Model file for the job. Use its own axes, mm. Face numbers are marked on the shaded views. A direction names the side the tool comes from. Round coordinates to 2 decimals unless told otherwise and drop trailing zeros. Write each loop counter-clockwise with the first axis right and the second up, starting at its lowest first coordinate (ties: lowest second). Pieces come first, ordered by that corner, then holes.
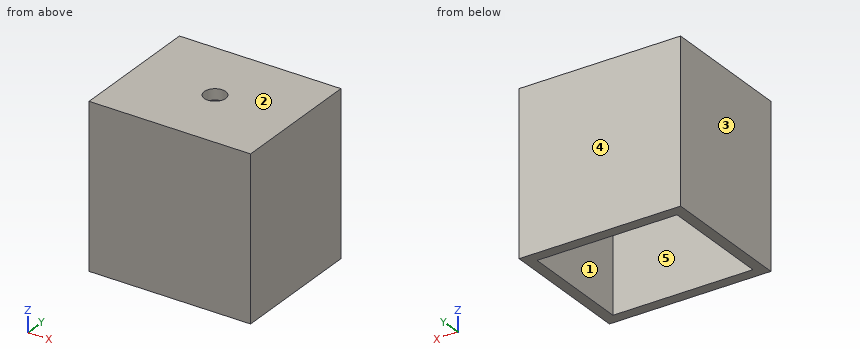
```python
from build123d import *

# Parameters (mm, degrees)
F0_W     = 15
F0_H     = 12.5
F1_DEPTH = 15
F2_T     = -1
F4_D     = 2


with BuildPart() as f1:
    # F0 (on Top) → F1 (new body)
    with BuildSketch(Plane.XY):
        Rectangle(F0_W, F0_H)
    extrude(amount=F1_DEPTH)

    # F2
    f2_openings = [f1.faces().sort_by_distance(p)[0] for p in [
        (0, 0, 0),
    ]]
    offset(amount=F2_T, openings=f2_openings)

    # F4 (through all)
    with Locations(Plane.XY.offset(15)):
        with Locations((0, 0)):
            Hole(F4_D / 2)


solid = f1.part
```
1) Wall check: probe 1 along Y at (x, z) = (3.75, 10.25); probe 2 along X at (y, z) = (-2.5, 7.75); probe 3 along Y at (x, z) = (0, 14.85). Give the ranges that are in metal, low to high.
2) Cut at B-B on z = 3. List the corners of the cut face in (x, y).
3) Pull direction X, two halves, no side cores. Call the marked faces 3, 4 and 5: released by +X, released by -X, zero draft, split by the parting line, or undercut.
4) Cut at A-A on y = 0. List the corners of the cut face in (x, z).
5) Flat gauge pin, fed straight in: pin 1 Ø3 at (x, y) = (-2, -1) entering from -Z. Where does the tip first touch, or does it go through?
6) Cut at C-C on x = 0. List the corners of the cut face in (y, z), and give its area (3 significant figures).
7) Cut at D-D on x = -3. List the corners of the cut face in (y, z), and give its area (3 significant figures).
8) Which spindle directions (+Z, -Z, +X, -X, +Y, -Y) get a long thin tool onto all of the face, cutting with end or side? Do the marked faces 1 and 2. Say none if no direction does.
Result sheet:
1. probe 1: y = -6.25 to -5.25, 5.25 to 6.25
1. probe 2: x = -7.5 to -6.5, 6.5 to 7.5
1. probe 3: y = -6.25 to -1, 1 to 6.25
2. outline: (-7.5, -6.25) - (7.5, -6.25) - (7.5, 6.25) - (-7.5, 6.25) - close; hole (-6.5, -5.25) - (6.5, -5.25) - (6.5, 5.25) - (-6.5, 5.25) - close
3. face 3: released by -X
3. face 4: zero draft
3. face 5: undercut
4. outline: (-7.5, 0) - (-6.5, 0) - (-6.5, 14) - (-1, 14) - (-1, 15) - (-7.5, 15) - close; (1, 14) - (6.5, 14) - (6.5, 0) - (7.5, 0) - (7.5, 15) - (1, 15) - close
5. pin 1: stops at z = 14
6. outline: (-6.25, 0) - (-5.25, 0) - (-5.25, 14) - (-1, 14) - (-1, 15) - (-6.25, 15) - close; (1, 14) - (5.25, 14) - (5.25, 0) - (6.25, 0) - (6.25, 15) - (1, 15) - close
6. area: 38.5 mm2
7. outline: (-6.25, 0) - (-5.25, 0) - (-5.25, 14) - (5.25, 14) - (5.25, 0) - (6.25, 0) - (6.25, 15) - (-6.25, 15) - close
7. area: 40.5 mm2
8. face 1: -Z
8. face 2: +Z, +X, -X, +Y, -Y
